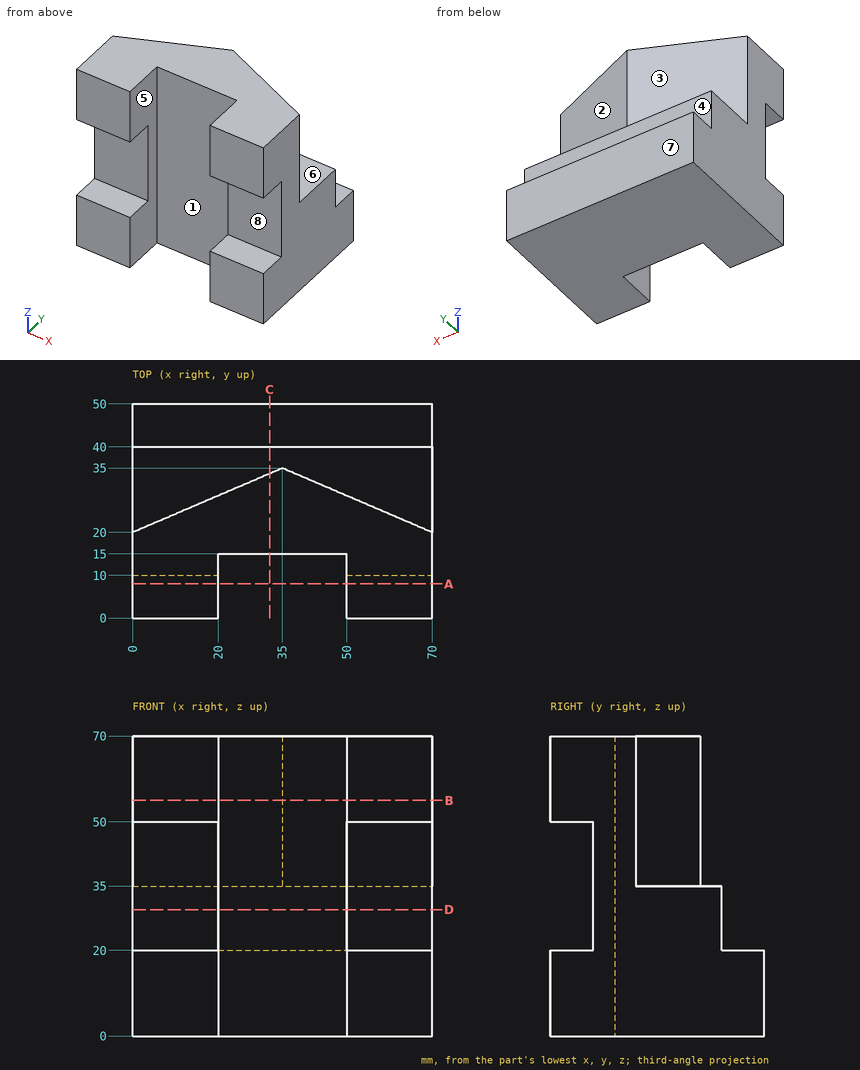
Geometry: see drawing. Coordinates: mm, zero at the bounding-box minimum. A direction names the side the tool comes from. Round coordinates to 2 decimals unless told otherwise and drop trailing zeros. Loops run counter-clockwise (first coordinate to the right, second up) from the corner with the lowest first, then second, coordinate; pieces in that order, holes last. Notation, with made-up numbers: (-38, 27) - (-2, 27) arc R32 cw to (-2, 61) - close; hole circle Ø6 at (72.25, 84). An arc over 180 degrees is marked (long way). One line per item, written item: value. Start each with the question number.
(1) Section B-B, the plane z = 55. Return loops of the section in (x, y).
(2) Section A-A, the plane y = 8. Return loops of the section in (x, z), plus the area to 3 significant figures.
(3) Draft query along X for the marked faces 1, 2, 3 and 4. Return one class per face: +X half, -X half, draft (parallel to the pull), parting line (faces both ways), or undercut.
(4) Ray query, line 1 (Z direction, x = 11.5, y = 6); line 2 (Y direction, x = 6.5, z = 33.5). Return the intervals inside material, ascending. Write a range as [from, to].
(5) Section D-D, the plane z = 29.5. Return loops of the section in (x, y), plus the area to 3 significant figures.
(6) Access query for the marked faces 5, 6, 7 and 8. Directions: +Z, -Z, +X, -X, +Y, -Y. A direction counts if a zero-diameter tool reaches every point of the face in a straight line with its end or side. Return the directions, or none.
(7) Contact query for flat-ended pins moving along their axis: P1, Ø10, axis at x = 64.5, z = 30.5, coming from the -Y side; P2, Ø16.5, axis at x = 42.5, z = 29.5, coming from the +Y side; P3, Ø24, axis at x = 37.5, z = 40, coming from the -Y side. Output: stop coordinate, or through.
(8) Section C-C, the plane x = 32. Return loops of the section in (y, z).
Results below:
1. outline: (0, 0) - (20, 0) - (20, 15) - (50, 15) - (50, 0) - (70, 0) - (70, 20) - (35, 35) - (0, 20) - close
2. outline: (0, 0) - (20, 0) - (20, 20) - (0, 20) - close; (0, 50) - (20, 50) - (20, 70) - (0, 70) - close; (50, 0) - (70, 0) - (70, 20) - (50, 20) - close; (50, 50) - (70, 50) - (70, 70) - (50, 70) - close
2. area: 1,600 mm^2
3. face 1: undercut
3. face 2: +X half
3. face 3: -X half
3. face 4: draft
4. line 1: [0, 20], [50, 70]
4. line 2: [10, 40]
5. outline: (0, 10) - (20, 10) - (20, 15) - (50, 15) - (50, 10) - (70, 10) - (70, 40) - (0, 40) - close
5. area: 1,950 mm^2
6. face 5: +Z, -Z, -Y
6. face 6: +Z, +Y
6. face 7: +Z, -Z, +X, -X, +Y
6. face 8: +X, -X, -Y
7. P1: y = 10
7. P2: y = 40
7. P3: y = 15
8. outline: (15, 0) - (50, 0) - (50, 20) - (40, 20) - (40, 35) - (33.71, 35) - (33.71, 70) - (15, 70) - close
